The model under review builds one solid part; all positions refer to its coordinate system, in mm. Give positions to 0.01 mm unless a question says otherwise; leave off trailing zeros. Order: outer loops, then holes, each group sorted by start corner. A loop starts at its lowest first (then second) coordinate and runs counter-clockwise, first axis right, second up.
```python
from build123d import *

# Parameters (mm, degrees)
F0_R     = 44.45
F0_R_2   = 25.4
F1_DEPTH = 7.62
F2_SIZE  = 5.08
F3_R     = 3.80999


# Not quite as in the source:
# - a fillet or chamfer is up to 0.001 mm smaller than in the source, because OpenCascade refuses the exact size


with BuildPart() as f1:
    # F0 (on Top) → F1 (new body)
    with BuildSketch(Plane.XY):
        Circle(F0_R)
        Circle(F0_R_2, mode=Mode.SUBTRACT)
    extrude(amount=F1_DEPTH)

    # F2
    f2_edges = [f1.edges().sort_by_distance(p)[0] for p in [
        (-25.4, 0, 7.62),
    ]]
    chamfer(f2_edges, length=F2_SIZE)

    # F3 (radius 3.81 in the source; OpenCascade refuses exactly that, so slightly less here)
    f3_edges = [f1.edges().sort_by_distance(p)[0] for p in [
        (44.45, 0, 3.81),
        (-44.45, 0, 0),
        (-44.45, 0, 7.62),
    ]]
    fillet(f3_edges, radius=F3_R)


solid = f1.part
```
1. To check wall thickness, follow line 1 (Y direction, x = 0, z = 1.8); line 2 (Y direction, x = -9.5, z = 4.75); line 3 (X direction, y = -18, z = 2.5). State the ranges of each line that lie inside material, in increasing order.
2. Insertion check: pin 1 (10 mm diameter, centred on x = -27, y = -4, fed in from +Z); pin 2 (1 mm diameter, centred on y = 12.5, z = 1, fed in from +X); pin 3 (1.5 mm diameter, centred on x = -17, z = 5, fed in from +Y); pin 4 (4 mm diameter, centred on y = -30, z = 1.5, fed in from -X). Each pin has a flat end and moves straight along its axis. Give the tip position at first contact, or say it passes through.
3. Draft analysis for pull direction Y (two halves, no side actions). For faces 1 (the conical face through (-5.58, -25.11, 2.86)), 2 (the flat face through (5.8, 30.3, 7.62)), state which applies: pulls with the +Y half, pulls with the -Y half, needs draft (parallel to the pull), parting line crosses it, or undercut.
4. Take a section at C-C (z = 5.75). Write out the cut boundary in (x, y).
Answer:
1. line 1: y = -43.88 to -25.4, 25.4 to 43.88
1. line 2: y = -43.3 to -25.92, 25.92 to 43.3
1. line 3: x = -40.39 to -17.92, 17.92 to 40.39
2. pin 1: stops at z = 7.62
2. pin 2: stops at x = 41.87
2. pin 3: stops at y = 41.24
2. pin 4: stops at x = -34
3. face 1: undercut
3. face 2: needs draft
4. outline: circle Ø87.84 at (0, 0); hole circle Ø57.22 at (0, 0)
